from build123d import *

# Parameters (mm, degrees)
SKETCH_1_W          = 50
SKETCH_1_H          = 50
SKETCH_1_R          = 1.35
EXTRUDE_1_DEPTH     = 3
EXTRUDE_START       = -3
SKETCH_2_W          = 50
SKETCH_2_H          = 115
SKETCH_2_R          = 1.35
SKETCH_2_R_2        = 1.55
EXTRUDE_2_DEPTH     = 3
CUT_EXTRUDE_1_DEPTH = 63.77141069
FILLET_2_R          = 2


with BuildPart() as part:
    # 草图1 → 凸台-拉伸1 (new body)
    with BuildSketch(Plane.XY):
        Rectangle(SKETCH_1_W, SKETCH_1_H)
        with Locations((18, 18)):
            Circle(SKETCH_1_R, mode=Mode.SUBTRACT)
        with Locations((-18, 18)):
            Circle(SKETCH_1_R, mode=Mode.SUBTRACT)
        with Locations((-18, -18)):
            Circle(SKETCH_1_R, mode=Mode.SUBTRACT)
        with Locations((18, -18)):
            Circle(SKETCH_1_R, mode=Mode.SUBTRACT)
    extrude(amount=EXTRUDE_1_DEPTH)

    # 草图2 → 凸台-拉伸2 (add)
    with BuildSketch(Plane.XY.offset(3).offset(EXTRUDE_START)):
        Rectangle(SKETCH_2_W, SKETCH_2_H)
        with Locations((18, 18)):
            Circle(SKETCH_2_R, mode=Mode.SUBTRACT)
        with Locations((18, -18)):
            Circle(SKETCH_2_R, mode=Mode.SUBTRACT)
        with Locations((-18, -18)):
            Circle(SKETCH_2_R, mode=Mode.SUBTRACT)
        with Locations((-18, 18)):
            Circle(SKETCH_2_R, mode=Mode.SUBTRACT)
        with Locations((-22, 54.5)):
            Circle(SKETCH_2_R_2, mode=Mode.SUBTRACT)
        with Locations((22, 54.5)):
            Circle(SKETCH_2_R_2, mode=Mode.SUBTRACT)
        with Locations((-22, -54.5)):
            Circle(SKETCH_2_R_2, mode=Mode.SUBTRACT)
        with Locations((22, -54.5)):
            Circle(SKETCH_2_R_2, mode=Mode.SUBTRACT)
    extrude(amount=EXTRUDE_2_DEPTH)

    # 草图8 → 切除-拉伸1 (cut, through all)
    with BuildSketch(Plane.XY.offset(3)):
        Polygon((12.910189133, -49.5), (0, -6.89637586), (-12.910189133, -49.5), align=None)
        Polygon((15, 42.60362414), (2.089810867, 0), (15, -42.60362414), align=None)
        Polygon((12.910189133, 49.5), (-12.910189133, 49.5), (0, 6.89637586), align=None)
        Polygon((-2.089810867, 0), (-15, 42.60362414), (-15, -42.60362414), align=None)
    extrude(amount=-CUT_EXTRUDE_1_DEPTH, mode=Mode.SUBTRACT)

    # 圆角2
    fillet_2_edges = [part.edges().sort_by_distance(p)[0] for p in [
        (25, 57.5, 1.5),
        (-25, -57.5, 1.5),
        (25, -57.5, 1.5),
        (-25, 57.5, 1.5),
        (0, 6.89637586, 1.5),
        (-12.910189133, 49.5, 1.5),
        (12.910189133, 49.5, 1.5),
        (2.089810867, 0, 1.5),
        (15, 42.60362414, 1.5),
        (15, -42.60362414, 1.5),
        (-15, -42.60362414, 1.5),
        (-15, 42.60362414, 1.5),
        (-2.089810867, 0, 1.5),
        (-12.910189133, -49.5, 1.5),
        (0, -6.89637586, 1.5),
        (12.910189133, -49.5, 1.5),
    ]]
    fillet(fillet_2_edges, radius=FILLET_2_R)


solid = part.part
Read the model definition and answer for the solid it produces. Units are mm, in the model's axes. A direction names the side the tool comes from. Round coordinates to 2 decimals unless told otherwise and drop trailing zeros. Write each loop counter-clockwise with the first axis right and the second up, starting at its lowest first coordinate (ties: lowest second). Pieces come first, ordered by that corner, then holes. Notation, with made-up numbers: M 0,-38.75 L 51,-38.75 A35 cw 51,-3.75 Z; hole C -3,18 d3. An arc over 180 degrees is marked long. Use a Markdown table: item, result.
1) For a pull along X with two mould halves and no side action, classify faces 3 (the cylindrical face through (-0.036, 11.793, 1.479)), 4 (the cylindrical face through (-24.43, 56.9, 1.52)), 5 (the flat face through (0, -57.5, 1)) as pulls with the +X half, pulls with the -X half, needs draft (parallel to the pull), parting line crosses it, or undercut.
Answers follow:
| item | result |
|---|---|
| face 3 | undercut |
| face 4 | pulls with the -X half |
| face 5 | needs draft |
2) The part is cut by section C-C (y = 6.5). Write down the section's boundary in (x, z), plus the area to 3 significant figures.
Answers follow:
| item | result |
|---|---|
| outline | M -25,0 L -15,0 L -15,3 L -25,3 Z; M -4.06,0 L 4.06,0 L 4.06,3 L -4.06,3 Z; M 15,0 L 25,0 L 25,3 L 15,3 Z |
| area | 84.4 mm2 |
3) Straight lines are drawn through the part: line 1 along Y through (x, z) = (18, 2.3); line 2 along Y through (x, z) = (-22, 2.15); line 3 along Y through (x, z) = (13, 1.7). For each, find the intervals that lie inside material, in ascending order. Write a range as [from, to].
Answers follow:
| item | result |
|---|---|
| line 1 | y = [-57.5, -19.35], [-16.65, 16.65], [19.35, 57.5] |
| line 2 | y = [-57.5, -56.05], [-52.95, 52.95], [56.05, 57.5] |
| line 3 | y = [-57.5, -31.11], [31.11, 57.5] |
4) A tool of negligible diameter and unlimited length cuts with its end or side. For faces 1 (the cylindrical face through (24.4, -56.93, 1.52)), 2 (the flat face through (-6.74, -15.34, 1.52)), from which of +Z, -Z, +X, -X, +Y, -Y can it reach the whole face along a straight path? Write none if from no direction.
Answers follow:
| item | result |
|---|---|
| face 1 | +Z, -Z, +X, -Y |
| face 2 | +Z, -Z |
5) The part is cut by section B-B (y = -18). Write down the section's boundary in (x, z).
Answers follow:
| item | result |
|---|---|
| outline | M -25,0 L -19.35,0 L -19.35,3 L -25,3 Z; M -16.65,0 L -15,0 L -15,3 L -16.65,3 Z; M -7.54,0 L -3.36,0 L -3.36,3 L -7.54,3 Z; M 3.36,0 L 7.54,0 L 7.54,3 L 3.36,3 Z; M 15,0 L 16.65,0 L 16.65,3 L 15,3 Z; M 19.35,0 L 25,0 L 25,3 L 19.35,3 Z |
6) The part is cut by section A-A (x = 18). Write down the section's boundary in (y, z).
Answers follow:
| item | result |
|---|---|
| outline | M -57.5,0 L -19.35,0 L -19.35,3 L -57.5,3 Z; M -16.65,0 L 16.65,0 L 16.65,3 L -16.65,3 Z; M 19.35,0 L 57.5,0 L 57.5,3 L 19.35,3 Z |
7) Flat-ended cylindrical pins translate along their axes: pin 1 (2.5 mm diameter, centred on x = -22, y = 54.5, fed in from +Z); pin 2 (5 mm diameter, centred on x = -22, y = -54.5, fed in from +Z). Find the tip coordinate at first contact, or state that the pin passes through.
Answers follow:
| item | result |
|---|---|
| pin 1 | passes through |
| pin 2 | stops at z = 3 |
8) The part is cut by section D-D (y = 21). Write down the section's boundary in (x, z), plus the area to 3 significant figures.
Answers follow:
| item | result |
|---|---|
| outline | M -25,0 L -15,0 L -15,3 L -25,3 Z; M -8.45,0 L -4.27,0 L -4.27,3 L -8.45,3 Z; M 4.27,0 L 8.45,0 L 8.45,3 L 4.27,3 Z; M 15,0 L 25,0 L 25,3 L 15,3 Z |
| area | 85.1 mm2 |
